Verification items for the finished model (mm, model axes). A direction names the side the tool comes from. Coordinates: 2 decimals unless noted, no trailing zeros. Write each loop counter-clockwise with the first axis right and the second up, starting at its lowest first coordinate (ties: lowest second). Pieces come first, ordered by that corner, then holes. Notation, with made-up numbers: (80.5, 81) -> (114.5, 81) arc R16 cw to (114.5, 92) -> close; hole circle Ø11 at (86.25, -40). An arc over 180 degrees is marked (long way). Answer in a Markdown table with one row per item.
```python
from build123d import *

# Parameters (mm, degrees)
PAD_DEPTH    = 2
PAD001_DEPTH = 4


with BuildPart() as part:
    # Sketch → Pad (new body)
    with BuildSketch(Plane.XY):
        with BuildLine():
            ThreePointArc((-50.500002, 40.499998), (-54.035539, 39.035536), (-55.50001, 35.500002))
            Line((-55.50001, -35.499998), (-55.50001, 35.500002))
            ThreePointArc((-55.50001, -35.499998), (-54.035544, -39.035532), (-50.50001, -40.499998))
            Line((50.49999, -40.499998), (-50.50001, -40.499998))
            ThreePointArc((50.49999, -40.499998), (54.035535, -39.03554), (55.50001, -35.500002))
            Line((55.50001, 35.499998), (55.50001, -35.500002))
            ThreePointArc((55.50001, 35.499998), (54.03554, 39.035536), (50.499998, 40.499998))
            Line((-50.500002, 40.499998), (50.499998, 40.499998))
        make_face()
    extrude(amount=PAD_DEPTH)

    # Sketch001 (on Face10 of Pad) → Pad001 (join)
    with BuildSketch(Plane.XY.offset(2)):
        with BuildLine():
            ThreePointArc((50.999999, 31.5), (49.68198, 34.68198), (46.500001, 36))
            Line((46.500001, 36), (-46.499999, 36))
            ThreePointArc((-46.499999, 36), (-49.68198, 34.68198), (-50.999999, 31.5))
            Line((-50.999999, 31.5), (-50.999999, -31.500002))
            ThreePointArc((-50.999999, -31.500002), (-49.681979, -34.681981), (-46.5, -36))
            Line((46.499999, -36), (-46.5, -36))
            ThreePointArc((46.499999, -36), (49.68198, -34.68198), (50.999999, -31.5))
            Line((50.999999, 31.5), (50.999999, -31.5))
        make_face()
        with BuildLine():
            ThreePointArc((-46.499999, 34), (-48.267766, 33.267767), (-48.999999, 31.5))
            Line((-48.999999, -31.500002), (-48.999999, 31.5))
            ThreePointArc((-48.999999, -31.500002), (-48.267765, -33.267769), (-46.499997, -34))
            Line((-46.499997, -34), (46.499999, -34))
            ThreePointArc((46.499999, -34), (48.267766, -33.267767), (48.999999, -31.5))
            Line((48.999999, -31.5), (48.999999, 31.499997))
            ThreePointArc((48.999999, 31.499997), (48.267765, 33.267768), (46.499994, 34))
            Line((-46.499999, 34), (46.499994, 34))
        make_face(mode=Mode.SUBTRACT)
    extrude(amount=PAD001_DEPTH)


solid = part.part
```
1. Thickness scan on line 1 (Y direction, x = 30.5, z = 3.1); line 2 (X direction, y = -30.5, z = 2.3); line 3 (Z direction, x = 32.5, y = -26.5). Record the ranges inside material, lowest first. Write a range as from..to.
Geometry says:
| item | result |
|---|---|
| line 1 | -36..-34, 34..36 |
| line 2 | -51..-49, 49..51 |
| line 3 | 0..2 |
2. Mould release check, pull along X, two halves, no side actions. Record for faces 5 (the flat face through (-49, 0, 4)), 6 (the flat face through (-1, 34, 4)), 7 (the cylindrical face through (-54, 39.07, 0.99)), 8 (the flat face through (-0.3, 36.2, 2)): released by +X, released by -X, zero draft, split by the parting line, or undercut.
Geometry says:
| item | result |
|---|---|
| face 5 | undercut |
| face 6 | undercut |
| face 7 | released by -X |
| face 8 | zero draft |
3. Section check B-B, the plane z = 4.1. Record the boundary of the cut face in (x, y), plus the area to 3 significant figures.
Geometry says:
| item | result |
|---|---|
| outline | (-51, -31.5) arc R4.5 ccw to (-46.5, -36) -> (46.5, -36) arc R4.5 ccw to (51, -31.5) -> (51, 31.5) arc R4.5 ccw to (46.5, 36) -> (-46.5, 36) arc R4.5 ccw to (-51, 31.5) -> close; hole (-49, -31.5) arc R2.5 ccw to (-46.5, -34) -> (46.5, -34) arc R2.5 ccw to (49, -31.5) -> (49, 31.5) arc R2.5 ccw to (46.5, 34) -> (-46.5, 34) arc R2.5 ccw to (-49, 31.5) -> close |
| area | 668 mm^2 |
4. Tool access check on faces 1 (the cylindrical face through (49.647, -34.717, 3.972)), 2 (the cylindrical face through (-49.647, 34.717, 3.972)), 3 (the flat face through (51, 0, 4)), 4 (the flat face through (1, 36, 4)). Record the directions out of +Z, -Z, +X, -X, +Y, -Y that give a thin tool (end or side, any length) a straight path to the whole face; none if there is none.
Geometry says:
| item | result |
|---|---|
| face 1 | +Z, +X, -Y |
| face 2 | +Z, -X, +Y |
| face 3 | +Z, +X, +Y, -Y |
| face 4 | +Z, +X, -X, +Y |
5. Section check C-C, the plane y = 2.5. Record the boundary of the cut face in (x, z), plus the area to 3 significant figures.
Geometry says:
| item | result |
|---|---|
| outline | (-55.5, 0) -> (55.5, 0) -> (55.5, 2) -> (51, 2) -> (51, 6) -> (49, 6) -> (49, 2) -> (-49, 2) -> (-49, 6) -> (-51, 6) -> (-51, 2) -> (-55.5, 2) -> close |
| area | 238 mm^2 |
6. Depth check by flat-ended pin: P1, Ø3, axis at y = -6.5, z = 5, coming from the +X side; P2, Ø1, axis at x = -13, z = 4, coming from the -Y side; P3, Ø6, axis at x = 34, y = 8, coming from the +Z side. Enter the tip coordinate at first touch or a pass-through.
Geometry says:
| item | result |
|---|---|
| P1 | x = 51 |
| P2 | y = -36 |
| P3 | z = 2 |
7. Section check A-A, the plane x = -0.5. Record the boundary of the cut face in (y, z), plus the area to 3 significant figures.
Geometry says:
| item | result |
|---|---|
| outline | (-40.5, 0) -> (40.5, 0) -> (40.5, 2) -> (36, 2) -> (36, 6) -> (34, 6) -> (34, 2) -> (-34, 2) -> (-34, 6) -> (-36, 6) -> (-36, 2) -> (-40.5, 2) -> close |
| area | 178 mm^2 |
